CAD build for the part. Positions are in the model's coordinates, mm. Round coordinates to 2 decimals unless told otherwise and drop trailing zeros. Loops run counter-clockwise (first coordinate to the right, second up) from the corner with the lowest first, then second, coordinate; pieces in that order, holes last. Notation, with made-up numbers: (65, 33.25) - (111, 33.25) arc R23 cw to (111, 71.25) - close; hole circle Ø1 at (-21.5, 52). An arc over 180 degrees is marked (long way). Use one line per item in the form item = value.
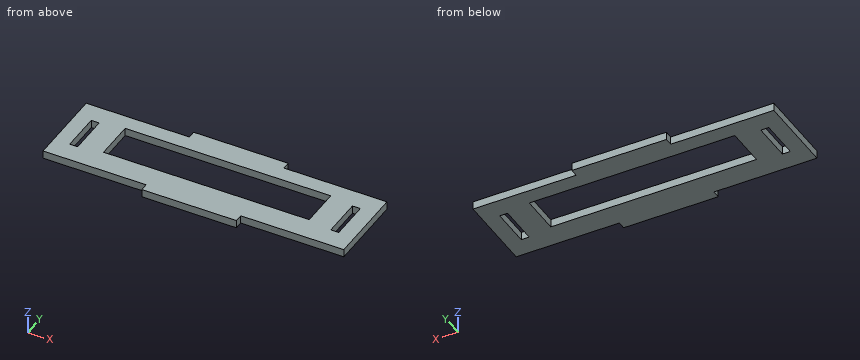
from build123d import *

# Parameters (mm, degrees)
SKETCH1_W           = 51.848
SKETCH1_H           = 10
SKETCH1_W_2         = 2
BOSS_EXTRUDE1_DEPTH = 2


with BuildPart() as part:
    # Sketch1 → Boss-Extrude1 (new body)
    with BuildSketch(Plane.XY):
        Polygon((0, 0), (24, 0), (24, -2), (47.848, -2), (47.848, 0), (71.848, 0), (73.848, 0), (73.848, 20), (71.848, 20), (47.848, 20), (47.848, 22), (24, 22), (24, 20), (0, 20), (-2, 20), (-2, 0), align=None)
        with Locations((35.924, 11)):
            Rectangle(SKETCH1_W, SKETCH1_H, mode=Mode.SUBTRACT)
        with Locations((3, 10)):
            Rectangle(SKETCH1_W_2, SKETCH1_H, mode=Mode.SUBTRACT)
        with Locations((68.848, 10)):
            Rectangle(SKETCH1_W_2, SKETCH1_H, mode=Mode.SUBTRACT)
    extrude(amount=BOSS_EXTRUDE1_DEPTH)


solid = part.part
1) Drill centre lines: probe 1 along X at (y, z) = (6.75, 0.4); probe 2 along Y at (x, z) = (3.5, 1.5); probe 3 along Y at (x, z) = (54.5, 0.4). Where is each one in solid material? Low to high.
Report:
probe_1 = -2 to 2, 4 to 10, 61.85 to 67.85, 69.85 to 73.85
probe_2 = 0 to 5, 15 to 20
probe_3 = 0 to 6, 16 to 20
2) Slice it at B-B (x = 28.5). Write the cut outline in (y, z), plus the area to 3 significant figures.
Report:
outline = (-2, 0) - (6, 0) - (6, 2) - (-2, 2) - close; (16, 0) - (22, 0) - (22, 2) - (16, 2) - close
area = 28.0 mm^2
3) Slice it at C-C (z = 0.75). Write the cut outline in (x, y).
Report:
outline = (-2, 0) - (24, 0) - (24, -2) - (47.85, -2) - (47.85, 0) - (73.85, 0) - (73.85, 20) - (47.85, 20) - (47.85, 22) - (24, 22) - (24, 20) - (-2, 20) - close; hole (2, 5) - (4, 5) - (4, 15) - (2, 15) - close; hole (10, 6) - (61.85, 6) - (61.85, 16) - (10, 16) - close; hole (67.85, 5) - (69.85, 5) - (69.85, 15) - (67.85, 15) - close
4) Flat gauge pins, fed straight in: pin 1 (0.6 mm diameter, centred on x = 63, z = 0.5, fed in from -Y); pin 2 (1 mm diameter, centred on x = 15.5, z = 1, fed in from +Y). Where does each tip first touch, or does it go through?
Report:
pin_1 = 0
pin_2 = 20
5) Slice it at A-A (y = 8.75). Write the cut outline in (x, z).
Report:
outline = (-2, 0) - (2, 0) - (2, 2) - (-2, 2) - close; (4, 0) - (10, 0) - (10, 2) - (4, 2) - close; (61.85, 0) - (67.85, 0) - (67.85, 2) - (61.85, 2) - close; (69.85, 0) - (73.85, 0) - (73.85, 2) - (69.85, 2) - close
